Input: part model. Units: mm. Frame: model coordinates. Round coordinates to 2 decimals unless told otherwise and drop trailing zeros. Loops run counter-clockwise (first coordinate to the right, second up) from the corner with the lowest first, then second, coordinate; pieces in that order, holes last. Notation, with made-up numbers: M -8,38.25 L -3,38.25 A16 cw -3,69.25 Z; hole C 83.5,-6 d6. An arc over 180 degrees is marked long. Return JSON: item names as keys, results as strings. Group by question number.
1) Section A-A (y = -7). Output: boundary loops of the cut face in (x, z).
2) Contact query for flat-ended pins moving along their axis: P1, Ø2.5, axis at x = 182.99, y = 126, coming from the -Z side; P2, Ø1, axis at y = 34.5, z = 0.5, coming from the +X side; P3, Ø1, axis at y = 37, z = 1, coming from the +X side. Output: stop coordinate, or through.
3) Material intervals for line 1 (Y direction, x = 160.5, z = 1.3); line 2 (Y direction, x = 71.5, z = 0.9); line 3 (X direction, y = 104.5, z = 1), sorted ascending. Write a range as from..to.
4) Section B-B (z = 1.5). Count the separate pieces of the cut face and the enclosed holes in it, plus the area to 3 significant figures.
from build123d import *

# Parameters (mm, degrees)
BOSS_EXTRUDE1_DEPTH = 2
SKETCH4_R           = 3.9998
SKETCH4_R_2         = 1.499925
SKETCH4_R_3         = 3.7498125
SKETCH4_R_4         = 10.99945
SKETCH4_R_5         = 4.99975
SKETCH4_R_6         = 3.999800521
CUT_EXTRUDE1_DEPTH  = 2


with BuildPart() as part:
    # Sketch3 → Boss-Extrude1 (new body)
    with BuildSketch(Plane.XY):
        with BuildLine():
            Line((-106.00519968, 144.943614194), (182.96308424, 145.197672799))
            add(Edge.make_bspline(
                [(214.06903129, 100.332253713), (217.202846332, 108.581551057), (216.384279944, 131.51380425), (195.382789786, 145.608716116), (182.96308424, 145.197672799)],
                knots=[0, 0, 0, 0, 0.416238876, 1, 1, 1, 1], degree=3))
            Line((214.06903129, 100.332253713), (171.900116679, -12))
            add(Edge.make_bspline(
                [(160.991950179, -19), (165.457889658, -19.068752161), (170.106996065, -16.09051608), (171.900116679, -12)],
                knots=[0, 0, 0, 0, 1, 1, 1, 1], degree=3))
            Line((160.991950179, -19), (-18.999049973, -19))
            add(Edge.make_bspline(
                [(-18.999049973, -19), (-23.419302443, -19.069581379), (-27.756029743, -16.362926839), (-29.701931061, -12.425576557)],
                knots=[0, 0, 0, 0, 1, 1, 1, 1], degree=3))
            Line((-29.701931061, -12.425576557), (-116.08546313, 126.611232779))
            add(Edge.make_bspline(
                [(-106.00519968, 144.943614194), (-112.924010598, 145.092654371), (-119.661868892, 137.031763828), (-117.348474018, 128.592298794), (-116.08546313, 126.611232779)],
                knots=[0, 0, 0, 0, 0.715346285, 1, 1, 1, 1], degree=3))
        make_face()
    extrude(amount=BOSS_EXTRUDE1_DEPTH)

    # Sketch4 → Cut-Extrude1 (cut)
    with BuildSketch(Plane.XY.offset(2)):
        with Locations((-105.9947, 133)):
            Circle(SKETCH4_R)
        with Locations((-78.996040132, 136.5)):
            Circle(SKETCH4_R_2)
        with Locations((-101.689209002, 118.598380963)):
            Circle(SKETCH4_R_2)
        with Locations((-91.134705429, 101.610600241)):
            Circle(SKETCH4_R_2)
        with Locations((-66.99665, 112)):
            Circle(SKETCH4_R_3)
        with Locations((-80.580283096, 84.622950275)):
            Circle(SKETCH4_R_2)
        with Locations((-5.9997, 133)):
            Circle(SKETCH4_R)
        with Locations((20.99895, 136.5)):
            Circle(SKETCH4_R_2)
        with Locations((20.99895, 96.5)):
            Circle(SKETCH4_R_2)
        with Locations((-18.99905, 96.5)):
            Circle(SKETCH4_R_2)
        with Locations((-58.99705, 96.5)):
            Circle(SKETCH4_R_2)
        with Locations((57.9971, 112)):
            Circle(SKETCH4_R)
        with Locations((60.99695, 96.5)):
            Circle(SKETCH4_R_2)
        with Locations((182.99085, 112)):
            Circle(SKETCH4_R_4)
        with Locations((182.99085, 126)):
            Circle(SKETCH4_R_2)
        with Locations((180.99095, 136.5)):
            Circle(SKETCH4_R_2)
        with Locations((120.99395, 136.5)):
            Circle(SKETCH4_R_2)
        with Locations((93.995220809, 133)):
            Circle(SKETCH4_R)
        with Locations((100.99495, 96.5)):
            Circle(SKETCH4_R_2)
        with Locations((140.99295, 96.5)):
            Circle(SKETCH4_R_2)
        with Locations((168.99155, 112)):
            Circle(SKETCH4_R_2)
        with Locations((196.99015, 112)):
            Circle(SKETCH4_R_2)
        with Locations((182.99085, 98)):
            Circle(SKETCH4_R_2)
        with Locations((205.322481122, 99.795751553)):
            Circle(SKETCH4_R_2)
        with Locations((198.324441471, 81.060193672)):
            Circle(SKETCH4_R_2)
        with Locations((150.99245, 64)):
            Circle(SKETCH4_R_5)
        with Locations((180.99095, 64)):
            Circle(SKETCH4_R_2)
        with Locations((191.32646769, 62.324812144)):
            Circle(SKETCH4_R_2)
        with Locations((120.99395, 64)):
            Circle(SKETCH4_R_2)
        with Locations((184.328557385, 43.589600555)):
            Circle(SKETCH4_R_2)
        with Locations((70.99645, 64)):
            Circle(SKETCH4_R_5)
        with Locations((20.99895, 64)):
            Circle(SKETCH4_R_2)
        with Locations((0.99995, 31.499992415)):
            Circle(SKETCH4_R_2)
        with Locations((40.99795, 31.499988622)):
            Circle(SKETCH4_R_2)
        with Locations((80.99595, 31.499985778)):
            Circle(SKETCH4_R_2)
        with Locations((120.99395, 31.499981037)):
            Circle(SKETCH4_R_2)
        with Locations((160.99195, 31.499978192)):
            Circle(SKETCH4_R_2)
        with Locations((177.330672341, 24.854456596)):
            Circle(SKETCH4_R_2)
        with Locations((-18.99905, 64)):
            Circle(SKETCH4_R_5)
        with Locations((-70.02547384, 67.634677545)):
            Circle(SKETCH4_R_2)
        with Locations((-58.99705, 64)):
            Circle(SKETCH4_R_2)
        with Locations((-59.470762984, 50.646563195)):
            Circle(SKETCH4_R_2)
        with Locations((-48.916261932, 33.658786529)):
            Circle(SKETCH4_R_2)
        with Locations((-38.99805, 31.499994311)):
            Circle(SKETCH4_R_2)
        with Locations((-38.361920415, 16.671266638)):
            Circle(SKETCH4_R_2)
        with Locations((20.99895, 0.5)):
            Circle(SKETCH4_R_2)
        with Locations((70.99645, -7)):
            Circle(SKETCH4_R_6)
        with Locations((160.99195, -7)):
            Circle(SKETCH4_R)
        with Locations((170.332531489, 6.118627774)):
            Circle(SKETCH4_R_2)
        with Locations((120.99395, 0.5)):
            Circle(SKETCH4_R_2)
        with BuildLine():
            Line((-18.99905, -3), (0.99995, -3))
            ThreePointArc((0.99995, -3), (4.997795472, -7.128933101), (0.749772406, -11))
            Line((0.749772406, -11), (-18.99905, -11))
            ThreePointArc((-18.99905, -11), (-22.99885, -7), (-18.99905, -3))
        make_face()
    extrude(amount=-CUT_EXTRUDE1_DEPTH, mode=Mode.SUBTRACT)


solid = part.part
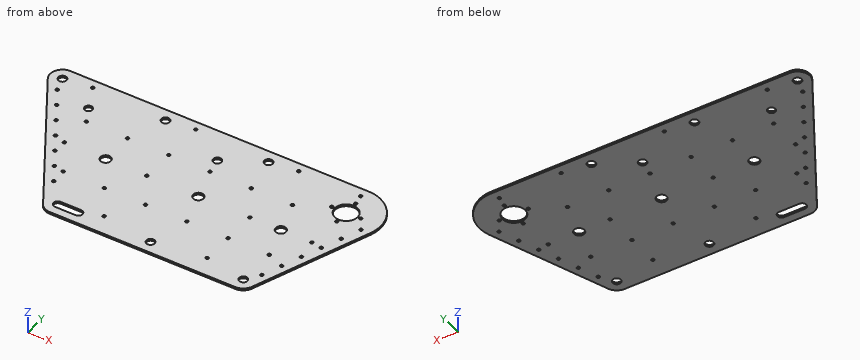
Returned:
{
 "1": {"outline": "M -33.07,0 L -23,0 L -23,2 L -33.07,2 Z; M 5,0 L 67,0 L 67,2 L 5,2 Z; M 75,0 L 156.99,0 L 156.99,2 L 75,2 Z; M 164.99,0 L 173.78,0 L 173.78,2 L 164.99,2 Z"},
 "2": {"P1": "passes through", "P2": "stops at x = 189.54", "P3": "stops at x = 190.48"},
 "3": {"line 1": "y = -19..-10.97, -3.03..30.08, 32.92..145.18", "line 2": "y = -19..-10.97, -3.03..59.03, 68.97..145.1", "line 3": "x = -102.35..174.94, 191.04..215.33"},
 "4": {"separate pieces": "1", "enclosed holes": "51", "area": "43,300 mm^2"}
}
